from build123d import *

# Parameters (mm, degrees)
CUT_EXTRUDE1_REACH = 135.082
SKETCH4_R          = 3.175


with BuildPart() as part:
    # Sketch1 → Revolve1 (revolve)
    with BuildSketch(Plane.XY, mode=Mode.PRIVATE) as revolve1_sk:
        Polygon((0, 47.6758), (79.9592, 74.9554), (79.9592, 75.223775525), (0, 47.944175525), align=None)
    revolve(revolve1_sk.sketch.rotate(Axis((0, 0, 0), (1, 0, 0)), 90), axis=Axis((0, 0, 0), (1, 0, 0)))

    # Sketch3 → Revolve2 (revolve)
    with BuildSketch(Plane.XY, mode=Mode.PRIVATE) as revolve2_sk:
        Polygon((0, 47.944175525), (3.175, 49.027387088), (3.175, 72.3138), (0, 72.3138), align=None)
    revolve(revolve2_sk.sketch.rotate(Axis((0, 0, 0), (1, 0, 0)), 90), axis=Axis((0, 0, 0), (1, 0, 0)))

    # Sketch4 → Cut-Extrude1 (cut, up to next)
    with BuildSketch(Plane.ZY, mode=Mode.PRIVATE) as cut_extrude1_sk1:
        with Locations((0, 67.31)):
            Circle(SKETCH4_R)
    cut_extrude1_tool1 = extrude(cut_extrude1_sk1.sketch, amount=-CUT_EXTRUDE1_REACH, mode=Mode.PRIVATE) & part.part
    # Sketch4 → Cut-Extrude1 (cut, up to next)
    with BuildSketch(Plane.ZY, mode=Mode.PRIVATE) as cut_extrude1_sk2:
        with Locations((20.799933891, 64.015614112)):
            Circle(SKETCH4_R)
    cut_extrude1_tool2 = extrude(cut_extrude1_sk2.sketch, amount=-CUT_EXTRUDE1_REACH, mode=Mode.PRIVATE) & part.part
    # Sketch4 → Cut-Extrude1 (cut, up to next)
    with BuildSketch(Plane.ZY, mode=Mode.PRIVATE) as cut_extrude1_sk3:
        with Locations((39.563825332, 54.454933891)):
            Circle(SKETCH4_R)
    cut_extrude1_tool3 = extrude(cut_extrude1_sk3.sketch, amount=-CUT_EXTRUDE1_REACH, mode=Mode.PRIVATE) & part.part
    # Sketch4 → Cut-Extrude1 (cut, up to next)
    with BuildSketch(Plane.ZY, mode=Mode.PRIVATE) as cut_extrude1_sk4:
        with Locations((54.454933891, 39.563825332)):
            Circle(SKETCH4_R)
    cut_extrude1_tool4 = extrude(cut_extrude1_sk4.sketch, amount=-CUT_EXTRUDE1_REACH, mode=Mode.PRIVATE) & part.part
    # Sketch4 → Cut-Extrude1 (cut, up to next)
    with BuildSketch(Plane.ZY, mode=Mode.PRIVATE) as cut_extrude1_sk5:
        with Locations((64.015614112, 20.799933891)):
            Circle(SKETCH4_R)
    cut_extrude1_tool5 = extrude(cut_extrude1_sk5.sketch, amount=-CUT_EXTRUDE1_REACH, mode=Mode.PRIVATE) & part.part
    # Sketch4 → Cut-Extrude1 (cut, up to next)
    with BuildSketch(Plane.ZY, mode=Mode.PRIVATE) as cut_extrude1_sk6:
        with Locations((67.31, 0)):
            Circle(SKETCH4_R)
    cut_extrude1_tool6 = extrude(cut_extrude1_sk6.sketch, amount=-CUT_EXTRUDE1_REACH, mode=Mode.PRIVATE) & part.part
    # Sketch4 → Cut-Extrude1 (cut, up to next)
    with BuildSketch(Plane.ZY, mode=Mode.PRIVATE) as cut_extrude1_sk7:
        with Locations((64.015614112, -20.799933891)):
            Circle(SKETCH4_R)
    cut_extrude1_tool7 = extrude(cut_extrude1_sk7.sketch, amount=-CUT_EXTRUDE1_REACH, mode=Mode.PRIVATE) & part.part
    # Sketch4 → Cut-Extrude1 (cut, up to next)
    with BuildSketch(Plane.ZY, mode=Mode.PRIVATE) as cut_extrude1_sk8:
        with Locations((54.454933891, -39.563825332)):
            Circle(SKETCH4_R)
    cut_extrude1_tool8 = extrude(cut_extrude1_sk8.sketch, amount=-CUT_EXTRUDE1_REACH, mode=Mode.PRIVATE) & part.part
    # Sketch4 → Cut-Extrude1 (cut, up to next)
    with BuildSketch(Plane.ZY, mode=Mode.PRIVATE) as cut_extrude1_sk9:
        with Locations((39.563825332, -54.454933891)):
            Circle(SKETCH4_R)
    cut_extrude1_tool9 = extrude(cut_extrude1_sk9.sketch, amount=-CUT_EXTRUDE1_REACH, mode=Mode.PRIVATE) & part.part
    # Sketch4 → Cut-Extrude1 (cut, up to next)
    with BuildSketch(Plane.ZY, mode=Mode.PRIVATE) as cut_extrude1_sk10:
        with Locations((20.799933891, -64.015614112)):
            Circle(SKETCH4_R)
    cut_extrude1_tool10 = extrude(cut_extrude1_sk10.sketch, amount=-CUT_EXTRUDE1_REACH, mode=Mode.PRIVATE) & part.part
    # Sketch4 → Cut-Extrude1 (cut, up to next)
    with BuildSketch(Plane.ZY, mode=Mode.PRIVATE) as cut_extrude1_sk11:
        with Locations((0, -67.31)):
            Circle(SKETCH4_R)
    cut_extrude1_tool11 = extrude(cut_extrude1_sk11.sketch, amount=-CUT_EXTRUDE1_REACH, mode=Mode.PRIVATE) & part.part
    # Sketch4 → Cut-Extrude1 (cut, up to next)
    with BuildSketch(Plane.ZY, mode=Mode.PRIVATE) as cut_extrude1_sk12:
        with Locations((-20.799933891, -64.015614112)):
            Circle(SKETCH4_R)
    cut_extrude1_tool12 = extrude(cut_extrude1_sk12.sketch, amount=-CUT_EXTRUDE1_REACH, mode=Mode.PRIVATE) & part.part
    # Sketch4 → Cut-Extrude1 (cut, up to next)
    with BuildSketch(Plane.ZY, mode=Mode.PRIVATE) as cut_extrude1_sk13:
        with Locations((-39.563825332, -54.454933891)):
            Circle(SKETCH4_R)
    cut_extrude1_tool13 = extrude(cut_extrude1_sk13.sketch, amount=-CUT_EXTRUDE1_REACH, mode=Mode.PRIVATE) & part.part
    # Sketch4 → Cut-Extrude1 (cut, up to next)
    with BuildSketch(Plane.ZY, mode=Mode.PRIVATE) as cut_extrude1_sk14:
        with Locations((-54.454933891, -39.563825332)):
            Circle(SKETCH4_R)
    cut_extrude1_tool14 = extrude(cut_extrude1_sk14.sketch, amount=-CUT_EXTRUDE1_REACH, mode=Mode.PRIVATE) & part.part
    # Sketch4 → Cut-Extrude1 (cut, up to next)
    with BuildSketch(Plane.ZY, mode=Mode.PRIVATE) as cut_extrude1_sk15:
        with Locations((-64.015614112, -20.799933891)):
            Circle(SKETCH4_R)
    cut_extrude1_tool15 = extrude(cut_extrude1_sk15.sketch, amount=-CUT_EXTRUDE1_REACH, mode=Mode.PRIVATE) & part.part
    # Sketch4 → Cut-Extrude1 (cut, up to next)
    with BuildSketch(Plane.ZY, mode=Mode.PRIVATE) as cut_extrude1_sk16:
        with Locations((-67.31, 0)):
            Circle(SKETCH4_R)
    cut_extrude1_tool16 = extrude(cut_extrude1_sk16.sketch, amount=-CUT_EXTRUDE1_REACH, mode=Mode.PRIVATE) & part.part
    # Sketch4 → Cut-Extrude1 (cut, up to next)
    with BuildSketch(Plane.ZY, mode=Mode.PRIVATE) as cut_extrude1_sk17:
        with Locations((-64.015614112, 20.799933891)):
            Circle(SKETCH4_R)
    cut_extrude1_tool17 = extrude(cut_extrude1_sk17.sketch, amount=-CUT_EXTRUDE1_REACH, mode=Mode.PRIVATE) & part.part
    # Sketch4 → Cut-Extrude1 (cut, up to next)
    with BuildSketch(Plane.ZY, mode=Mode.PRIVATE) as cut_extrude1_sk18:
        with Locations((-54.454933891, 39.563825332)):
            Circle(SKETCH4_R)
    cut_extrude1_tool18 = extrude(cut_extrude1_sk18.sketch, amount=-CUT_EXTRUDE1_REACH, mode=Mode.PRIVATE) & part.part
    # Sketch4 → Cut-Extrude1 (cut, up to next)
    with BuildSketch(Plane.ZY, mode=Mode.PRIVATE) as cut_extrude1_sk19:
        with Locations((-39.563825332, 54.454933891)):
            Circle(SKETCH4_R)
    cut_extrude1_tool19 = extrude(cut_extrude1_sk19.sketch, amount=-CUT_EXTRUDE1_REACH, mode=Mode.PRIVATE) & part.part
    # Sketch4 → Cut-Extrude1 (cut, up to next)
    with BuildSketch(Plane.ZY, mode=Mode.PRIVATE) as cut_extrude1_sk20:
        with Locations((-20.799933891, 64.015614112)):
            Circle(SKETCH4_R)
    cut_extrude1_tool20 = extrude(cut_extrude1_sk20.sketch, amount=-CUT_EXTRUDE1_REACH, mode=Mode.PRIVATE) & part.part
    add(cut_extrude1_tool1.solids().sort_by_distance((0, 67.31, 0))[0], mode=Mode.SUBTRACT)
    add(cut_extrude1_tool2.solids().sort_by_distance((0, 64.015614, 20.799934))[0], mode=Mode.SUBTRACT)
    add(cut_extrude1_tool3.solids().sort_by_distance((0, 54.454934, 39.563825))[0], mode=Mode.SUBTRACT)
    add(cut_extrude1_tool4.solids().sort_by_distance((0, 39.563825, 54.454934))[0], mode=Mode.SUBTRACT)
    add(cut_extrude1_tool5.solids().sort_by_distance((0, 20.799934, 64.015614))[0], mode=Mode.SUBTRACT)
    add(cut_extrude1_tool6.solids().sort_by_distance((0, 0, 67.31))[0], mode=Mode.SUBTRACT)
    add(cut_extrude1_tool7.solids().sort_by_distance((0, -20.799934, 64.015614))[0], mode=Mode.SUBTRACT)
    add(cut_extrude1_tool8.solids().sort_by_distance((0, -39.563825, 54.454934))[0], mode=Mode.SUBTRACT)
    add(cut_extrude1_tool9.solids().sort_by_distance((0, -54.454934, 39.563825))[0], mode=Mode.SUBTRACT)
    add(cut_extrude1_tool10.solids().sort_by_distance((0, -64.015614, 20.799934))[0], mode=Mode.SUBTRACT)
    add(cut_extrude1_tool11.solids().sort_by_distance((0, -67.31, 0))[0], mode=Mode.SUBTRACT)
    add(cut_extrude1_tool12.solids().sort_by_distance((0, -64.015614, -20.799934))[0], mode=Mode.SUBTRACT)
    add(cut_extrude1_tool13.solids().sort_by_distance((0, -54.454934, -39.563825))[0], mode=Mode.SUBTRACT)
    add(cut_extrude1_tool14.solids().sort_by_distance((0, -39.563825, -54.454934))[0], mode=Mode.SUBTRACT)
    add(cut_extrude1_tool15.solids().sort_by_distance((0, -20.799934, -64.015614))[0], mode=Mode.SUBTRACT)
    add(cut_extrude1_tool16.solids().sort_by_distance((0, 0, -67.31))[0], mode=Mode.SUBTRACT)
    add(cut_extrude1_tool17.solids().sort_by_distance((0, 20.799934, -64.015614))[0], mode=Mode.SUBTRACT)
    add(cut_extrude1_tool18.solids().sort_by_distance((0, 39.563825, -54.454934))[0], mode=Mode.SUBTRACT)
    add(cut_extrude1_tool19.solids().sort_by_distance((0, 54.454934, -39.563825))[0], mode=Mode.SUBTRACT)
    add(cut_extrude1_tool20.solids().sort_by_distance((0, 64.015614, -20.799934))[0], mode=Mode.SUBTRACT)


solid = part.part
The listing builds one solid part. Answer for the finished solid, in the listing's coordinates (mm). A direction names the side the tool comes from. Round coordinates to 2 decimals unless told otherwise and drop trailing zeros. Write each loop counter-clockwise with the first axis right and the second up, starting at its lowest first coordinate (ties: lowest second). Pieces come first, ordered by that corner, then holes. Notation, with made-up numbers: M -18.5,33 L -3.5,33 A30 ccw -3.5,68 Z; hole C 53,11.25 d11. An arc over 180 degrees is marked long. Write each question's results on one line, items separated by ' | '. Start each with the question number.
Item 1: A cutting plane is placed at A-A on z = 0. Write down the section's boundary in (x, y) (3 decimals), and give its area (3 significant figures).
Item 2: For a pull along Y with two mould halves and no side action, classify faces 3 (the face through (1.565, -21.721, 68.974)), 4 (the face through (1.565, -19.846, -60.987)), 5 (the face through (0, 47, 15)) as pulls with the +Y half, pulls with the -Y half, needs draft (parallel to the pull), parting line crosses it, or undercut.
Item 3: A cutting plane is placed at D-D on x = 49. Write down the section's boundary in (y, z).
Item 4: Straight lines are drawn through the part: L1, parallel to Y at x = 35, z = -31; L2, parallel to X at y = -34, z = 53 (3 decimals); L3, parallel to Y at x = 47, z = 59. For each, find the intervals that lie inside material, in ascending order. Write a range as [from, to].
Item 5: For faces 1 (the face through (22.771, -16.654, 52.884)), 2 (the face through (1.57, 54.59, 36.39)), determine the directions among +Z, -Z, +X, -X, +Y, -Y from which every point of the face is accessible in a straight line to the end or side of a thin tool.
Item 6: Flat-ended cylindrical pins translate along their axes: pin 1 Ø1 at (x, y) = (71.5, -10) entering from +Z; pin 2 Ø5 at (x, y) = (45.5, -58) entering from -Z; pin 3 Ø6 at (x, y) = (50.5, 30.5) entering from -Z. Find the tip coordinate at first contact, or state that the pin passes through.
Check sheet entries:
1) outline: M 0,-72.314 L 3.175,-72.314 L 3.175,-70.485 L 0,-70.485 Z; M 0,-64.135 L 3.175,-64.135 L 3.175,-49.027 L 79.959,-75.224 L 79.959,-74.955 L 0,-47.676 Z; M 0,47.676 L 79.959,74.955 L 79.959,75.224 L 3.175,49.027 L 3.175,64.135 L 0,64.135 Z; M 0,70.485 L 3.175,70.485 L 3.175,72.314 L 0,72.314 Z | area: 154 mm²
2) face 3: parting line crosses it | face 4: undercut | face 5: needs draft
3) outline: C 0,0 d129.32; hole C 0,0 d128.79
4) L1: [-51.24, -50.92], [50.92, 51.24] | L2: [0, 3.175], [44.037, 44.824] | L3: [-24.75, -24.04], [24.04, 24.75]
5) face 1: +X | face 2: -X
6) pin 1: z = 71.83 | pin 2: z = -31.12 | pin 3: z = -59.48
